```python
from build123d import *

# Parameters (mm, degrees)
SKETCH1_W           = 135
SKETCH1_H           = 68
BOSS_EXTRUDE1_DEPTH = 3
SKETCH2_W           = 3
SKETCH2_H           = 12.2
SKETCH2_H_2         = 28
CUT_EXTRUDE1_DEPTH  = 3
SKETCH3_W           = 21.75
SKETCH3_H           = 3
CUT_EXTRUDE2_DEPTH  = 3
SKETCH4_W           = 13.5
SKETCH4_H           = 14.5
BOSS_EXTRUDE2_DEPTH = 45


with BuildPart() as part:
    # Sketch1 → Boss-Extrude1 (new body)
    with BuildSketch(Plane(origin=(0, 0, 0), x_dir=(1, 0, 0), z_dir=(0, 1, 0))):
        Rectangle(SKETCH1_W, SKETCH1_H)
    extrude(amount=BOSS_EXTRUDE1_DEPTH)

    # Sketch2 → Cut-Extrude1 (cut)
    with BuildSketch(Plane(origin=(0, 3, 0), x_dir=(1, 0, 0), z_dir=(0, 1, 0))):
        with Locations((-66, 27.9)):
            Rectangle(SKETCH2_W, SKETCH2_H)
        with Locations((-66, 0)):
            Rectangle(SKETCH2_W, SKETCH2_H_2)
        with Locations((-66, -27.9)):
            Rectangle(SKETCH2_W, SKETCH2_H)
    cut_extrude1 = extrude(amount=-CUT_EXTRUDE1_DEPTH, mode=Mode.SUBTRACT)

    # Mirror1: Cut-Extrude1 across plane
    add(cut_extrude1.mirror(Plane(origin=(0, 0, 0), x_dir=(0, 0, 1), z_dir=(1, 0, 0))), mode=Mode.SUBTRACT)

    # Sketch3 → Cut-Extrude2 (cut)
    with BuildSketch(Plane(origin=(0, 3, 0), x_dir=(1, 0, 0), z_dir=(0, 1, 0))):
        with Locations((-53.625, 32.5)):
            Rectangle(SKETCH3_W, SKETCH3_H)
        Polygon((28.75, 34), (-28.75, 34), (-28.75, 30.671368382), (28.75, 31), align=None)
        with Locations((53.625, 32.5)):
            Rectangle(SKETCH3_W, SKETCH3_H)
    cut_extrude2 = extrude(amount=-CUT_EXTRUDE2_DEPTH, mode=Mode.SUBTRACT)

    # Mirror2: Cut-Extrude2 across plane
    add(cut_extrude2.mirror(Plane.XY), mode=Mode.SUBTRACT)

    # Sketch4 → Boss-Extrude2 (add)
    with BuildSketch(Plane(origin=(0, 3, 0), x_dir=(1, 0, 0), z_dir=(0, 1, 0))):
        with Locations((50.39, 14.85)):
            Rectangle(SKETCH4_W, SKETCH4_H)
    extrude(amount=BOSS_EXTRUDE2_DEPTH)


solid = part.part
```
Input: part model. Units: mm. Frame: model coordinates. A direction names the side the tool comes from. Give positions to 0.01 mm unless a question says otherwise; leave off trailing zeros. Order: outer loops, then holes, each group sorted by start corner. A loop starts at its lowest first (then second) coordinate and runs counter-clockwise, first axis right, second up. Notation, with made-up numbers: M 15.25,3.5 L 52.25,3.5 A15 ccw 52.25,18.5 Z; hole C -11,-38.75 d2. An arc over 180 degrees is marked long. One line per question, with ' | ' between items. Start each with the question number.
1. Access query for faces 1 (the face through (64.5, 2, 0)), 2 (the face through (-66, 2, 14)), 3 (the face through (66, 2, -21.8)), 4 (the face through (64.5, 2, 26)). Directions: +Z, -Z, +X, -X, +Y, -Y. A direction counts if a zero-diameter tool reaches every point of the face in a straight line with its end or side. Return the directions, or none.
2. First-contact query: pin 1 Ø11.5 at (y, z) = (35, -16.5) entering from +X; pin 2 Ø0.9 at (y, z) = (1.5, 32) entering from -X; pin 3 Ø4 at (x, y) = (48, 35.5) entering from -Z. Flat tips, straight axial feed; report the tip coordinate or a pass-through.
3. Section query D-D (z = 18). Return the cut outline in (x, y), and give its area (3 significant figures).
4. Section query C-C (y = 29.5). Return the cut outline in (x, z), and give its area (3 significant figures).
5. Section query A-A (x = 51). Return the cut outline in (y, z).
6. Section query B-B (z = -15.5). Return the cut outline in (x, y), and give its area (3 significant figures).
7. Pull-direction query (X, two-part tool) for faces 5 (the face through (-54, 2, 31)), 6 (the face through (28.75, 2, -32)), 7 (the face through (43.64, 25, -15)); classes: released by +X, released by -X, zero draft, split by the parting line, or undercut.
8. Material intervals for probe 1 along Y at (x, z) = (47.5, -24); probe 2 along Z at (x, y) = (48, 2); probe 3 along X at (y, z) = (2, 30), sorted ascending. Write a range as [from, to].
Here are the results:
1) face 1: +X, +Y, -Y | face 2: -X, +Y, -Y | face 3: -Z, +X, +Y, -Y | face 4: +Z, +X, +Y, -Y
2) pin 1: x = 57.14 | pin 2: x = -42.75 | pin 3: z = -22.1
3) outline: M -67.5,0 L 67.5,0 L 67.5,3 L -67.5,3 Z | area: 405 mm²
4) outline: M 43.64,-22.1 L 57.14,-22.1 L 57.14,-7.6 L 43.64,-7.6 Z | area: 196 mm²
5) outline: M 0,-31 L 3,-31 L 3,-22.1 L 48,-22.1 L 48,-7.6 L 3,-7.6 L 3,31 L 0,31 Z
6) outline: M -67.5,0 L 67.5,0 L 67.5,3 L 57.14,3 L 57.14,48 L 43.64,48 L 43.64,3 L -67.5,3 Z | area: 1,010 mm²
7) face 5: zero draft | face 6: undercut | face 7: released by -X
8) probe 1: [0, 3] | probe 2: [-31, 31] | probe 3: [-64.5, 64.5]
